Check sheet for the modelled part. Datum: model origin and axes. Units: mm. Give positions to 0.01 mm unless a question says otherwise; leave off trailing zeros. Order: outer loops, then holes, each group sorted by start corner. A loop starts at its lowest first (then second) coordinate and runs counter-clockwise, first axis right, second up. Notation, with made-up numbers: (-25.75, -13) -> (-1.75, -13) arc R22 cw to (-1.75, -5) -> close; hole circle Ø1 at (41.5, 17.5). An arc over 180 degrees is marked (long way). Answer in a Markdown table with one row per item. Add a question column.
(1) Go/stop test with flat-tipped pins: pin 1 (1.5 mm diameter, centred on x = 1, z = 2.5, fed in from -Y); pin 2 (1 mm diameter, centred on y = -43.5, z = 0.5, fed in from -X). Record where each tip stops, or that it passes through.
(2) Cross-section at A-A (y = 0). State how many separate pieces and enclosed holes the cut face has, then the cut area to 3 significant figures.
(3) Cross-section at B-B (x = -8). Record the cut outline in (y, z) (3 decimals), then the cut area to 3 significant figures.
(4) Cross-section at D-D (y = -58.5). Record the cut outline in (x, z) (3 decimals).
(5) Thickness scan on L1, parallel to Y at x = 0, z = 0.95; L2, parallel to Y at x = -24, z = 0.4; L3, parallel to X at y = 44, z = 1.6. Record the ranges inside material, lowest first. Write a range as [from, to].
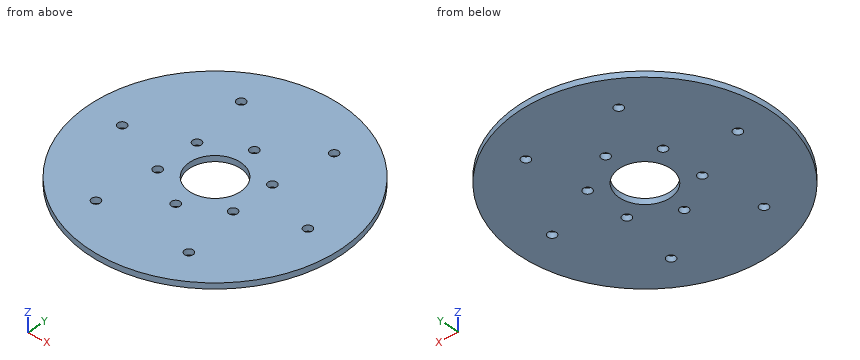
```python
from build123d import *

# Parameters (mm, degrees)
F0_R            = 69.85
F0_R_2          = 14.1605
F1_DEPTH        = 3.175
F2_R            = 2.3622
F3_DEPTH        = 3.176
F3_COPIES_COUNT = 6


# Not quite as in the source:
# - a pattern or mirror of a feature is missing from the dataset's text; its kind, count and spacing are read off the source's solid


with BuildPart() as f1:
    # F0 (on Top) → F1 (new body)
    with BuildSketch(Plane.XY):
        Circle(F0_R)
        Circle(F0_R_2, mode=Mode.SUBTRACT)
    extrude(amount=F1_DEPTH)

    # F2 (on face) → F3 (cut, through all)
    with BuildSketch(Plane.XY.offset(3.175)):
        with Locations((0, 23.8125)):
            Circle(F2_R)
        with Locations((25.4, 43.9940905122)):
            Circle(F2_R)
    f3 = extrude(amount=-F3_DEPTH, mode=Mode.SUBTRACT)

    # F3_copies: F3 ×6 about axis
    f3_copies_axis = Axis((0, 0, 0), (0, 0, 1))
    for i in range(1, F3_COPIES_COUNT):
        add(f3.rotate(f3_copies_axis, i * 360 / F3_COPIES_COUNT), mode=Mode.SUBTRACT)


solid = f1.part
```
Answer below:
| question | item | result |
|---|---|---|
| 1 | pin 1 | stops at y = -69.85 |
| 1 | pin 2 | stops at x = -55.05 |
| 2 | separate pieces | 4 |
| 2 | enclosed holes | 0 |
| 2 | area | 324 mm² |
| 3 | outline | (-69.39, 0) -> (-11.684, 0) -> (-11.684, 3.175) -> (-69.39, 3.175) -> close; (11.684, 0) -> (69.39, 0) -> (69.39, 3.175) -> (11.684, 3.175) -> close |
| 3 | area | 366 mm² |
| 4 | outline | (-38.168, 0) -> (38.168, 0) -> (38.168, 3.175) -> (-38.168, 3.175) -> close |
| 5 | L1 | y = [-69.85, -26.17], [-21.45, -14.16], [14.16, 21.45], [26.17, 69.85] |
| 5 | L2 | y = [-65.6, -45.9], [-42.09, 42.09], [45.9, 65.6] |
| 5 | L3 | x = [-54.25, -27.76], [-23.04, 23.04], [27.76, 54.25] |
